Model file for the job. Use its own axes, mm. A direction names the side the tool comes from. Coordinates: 2 decimals unless noted, no trailing zeros. Write each loop counter-clockwise with the first axis right and the second up, starting at its lowest first coordinate (ties: lowest second). Pieces come first, ordered by that corner, then holes. Notation, with made-up numbers: (43.25, 53.25) - (54.25, 53.25) arc R23 ccw to (54.25, 86.25) - close; hole circle Ø9 at (10, 49). An arc over 180 degrees is marked (long way). Put each result on its own line as item: value. Start each with the question number.
1. Drop flat-ended pins along their axis: P1, Ø6.5, axis at x = -0.5, z = -3, coming from the -Y side; P2, Ø5, axis at x = 8, y = 10, coming from the -Z side; P3, Ø1, axis at x = -7.5, z = -1, coming from the -Y side. Give the stop position or say it passes through.
2. Saw through at A-A, the plane z = -2.75. Write the cut outline in (x, y), plus the area to 3 significant figures.
3. Which spindle directions (+Z, -Z, +X, -X, +Y, -Y) get a long thin tool onto all of the face, cutting with end or side? Do faces 1 (the face through (0, 0, 0)), 2 (the face through (0.2, -24, -6.5)), 3 (the face through (0, 23.5, 1)), 4 (the face through (15, -2, 2)), 5 (the face through (0, -23.5, 0)). Say none if no direction does.
4. Drill centre lines: L1, parallel to Y at x = -11, z = -5; L2, parallel to Y at x = 3.5, z = -0.5; L3, parallel to Z at x = -5.5, y = -20. Where is each one in solid material? Low to high. Write a range as from..to.
5. Saw through at C-C, the plane y = -10. Write the cut outline in (x, z), plus the area to 3 significant figures.
6. Saw through at D-D, the plane z = -5.5. Write the cut outline in (x, y).
7. Saw through at B-B, the plane x = -10.5. Write the cut outline in (y, z), plus the area to 3 significant figures.
```python
from build123d import *

# Parameters (mm, degrees)
SKETCH_1_W      = 30
SKETCH_1_H      = 47
EXTRUDE_1_DEPTH = 3
SKETCH_2_W      = 30
SKETCH_2_H      = 1
EXTRUDE_2_DEPTH = 8
EXTRUDE_3_DEPTH = 30


with BuildPart() as part:
    # 草图1 → 凸台-拉伸1 (new body)
    with BuildSketch(Plane.XY):
        Rectangle(SKETCH_1_W, SKETCH_1_H)
    extrude(amount=EXTRUDE_1_DEPTH)

    # 草图2 → 凸台-拉伸2 (add)
    with BuildSketch(Plane(origin=(0, 0, 0), x_dir=(-1, 0, 0), z_dir=(0, 0, -1))):
        with Locations((0, 23)):
            Rectangle(SKETCH_2_W, SKETCH_2_H)
        with Locations((0, -23)):
            Rectangle(SKETCH_2_W, SKETCH_2_H)
    extrude(amount=EXTRUDE_2_DEPTH)

    # 草图3 → 凸台-拉伸3 (add, through all)
    with BuildSketch(Plane(origin=(15, 0, 0), x_dir=(0, 0, -1), z_dir=(1, 0, 0))):
        Polygon((2, 23.5), (8, 23.5), (5, 24.5), align=None)
        Polygon((8, -23.5), (2, -23.5), (5, -24.5), align=None)
    extrude(amount=-EXTRUDE_3_DEPTH)


solid = part.part
```
Final values:
1. P1: stops at y = -24.5
1. P2: stops at z = 0
1. P3: stops at y = -23.5
2. outline: (-15, -23.75) - (15, -23.75) - (15, -22.5) - (-15, -22.5) - close; (-15, 22.5) - (15, 22.5) - (15, 23.75) - (-15, 23.75) - close
2. area: 75.0 mm²
3. face 1: -Z, +X, -X
3. face 2: -Z, +X, -X, -Y
3. face 3: +Z, +X, -X, +Y
3. face 4: +Z, -Z, +X, +Y, -Y
3. face 5: +Z, +X, -X, -Y
4. L1: y = -24.5..-22.5, 22.5..24.5
4. L2: y = -23.5..-22.5, 22.5..23.5
4. L3: z = 0..3
5. outline: (-15, 0) - (15, 0) - (15, 3) - (-15, 3) - close
5. area: 90.0 mm²
6. outline: (-15, -24.33) - (15, -24.33) - (15, -22.5) - (-15, -22.5) - close; (-15, 22.5) - (15, 22.5) - (15, 24.33) - (-15, 24.33) - close
7. outline: (-24.5, -5) - (-23.5, -8) - (-22.5, -8) - (-22.5, 0) - (22.5, 0) - (22.5, -8) - (23.5, -8) - (24.5, -5) - (23.5, -2) - (23.5, 3) - (-23.5, 3) - (-23.5, -2) - close
7. area: 163 mm²
